Could you check a few things on this model? Use its own coordinates, in mm. Round coordinates to 2 decimals unless told otherwise and drop trailing zeros. Order: outer loops, then holes, each group sorted by start corner. A loop starts at its lowest first (then second) coordinate and runs counter-clockwise, first axis right, second up. Notation, with made-up numbers: (85, 22) - (118, 22) arc R12 ccw to (118, 38) - close; hole circle Ø2 at (43, 76). An arc over 180 degrees is marked (long way). Return JSON: item names as keys, results as strings. Group by question number.
from build123d import *

# Parameters (mm, degrees)
SKETCH_1_W             = 70
SKETCH_1_H             = 310
EXTRUDE_1_DEPTH        = 12
SKETCH_2_R             = 13
CUT_EXTRUDE_1_DEPTH    = 160.354949719
PATTERN_LINEAR_1_COUNT = 4
PATTERN_LINEAR_1_PITCH = 80


with BuildPart() as part:
    # 草图1 → 凸台-拉伸1 (new body)
    with BuildSketch(Plane.XY):
        Rectangle(SKETCH_1_W, SKETCH_1_H)
    extrude(amount=EXTRUDE_1_DEPTH)

    # 草图2 → 切除-拉伸1 (cut, through all)
    with BuildSketch(Plane.XY.offset(12)):
        with Locations((0, 120)):
            Circle(SKETCH_2_R)
    cut_extrude_1 = extrude(amount=-CUT_EXTRUDE_1_DEPTH, mode=Mode.SUBTRACT)

    # 阵列(线性)1: 切除-拉伸1 ×4
    with Locations(*[(0, -i * PATTERN_LINEAR_1_PITCH, 0) for i in range(1, PATTERN_LINEAR_1_COUNT)]):
        add(cut_extrude_1, mode=Mode.SUBTRACT)


solid = part.part
1) If I drill on line 1 along Y through (x, z) = (0, 9.5); line 2 along Y through (x, z) = (3.5, 5.5); line 3 along X through (y, z) = (113.5, 10.75), over which ranges is the centre line in solid material (lowest first)? Write a range as from..to.
2) I want a section at C-C, the plane z = 10. List the corners of the cut face in (x, y) for me.
3) We'd pull the mould along X, two halves only. Please class faces 1 (the flat face through (0, -155, 6)), 2 (the cylindrical face through (-2.82, -132.69, 6.08)), 3 (the flat face through (35, -2, 6)): +X half, -X half, draft (parallel to the pull), parting line (faces both ways), or undercut.
4) I want a section at A-A, the plane y = 40. List the corners of the cut face in (x, z) for me.
5) I want a section at B-B, the plane x = 0. List the corners of the cut face in (y, z) for me, plus the area to 3 significant figures.
Outcome:
{
 "1": {"line 1": "-155..-133, -107..-53, -27..27, 53..107, 133..155", "line 2": "-155..-132.52, -107.48..-52.52, -27.48..27.48, 52.52..107.48, 132.52..155", "line 3": "-35..-11.26, 11.26..35"},
 "2": {"outline": "(-35, -155) - (35, -155) - (35, 155) - (-35, 155) - close; hole circle Ø26 at (0, -120); hole circle Ø26 at (0, -40); hole circle Ø26 at (0, 40); hole circle Ø26 at (0, 120)"},
 "3": {"face 1": "draft", "face 2": "undercut", "face 3": "+X half"},
 "4": {"outline": "(-35, 0) - (-13, 0) - (-13, 12) - (-35, 12) - close; (13, 0) - (35, 0) - (35, 12) - (13, 12) - close"},
 "5": {"outline": "(-155, 0) - (-133, 0) - (-133, 12) - (-155, 12) - close; (-107, 0) - (-53, 0) - (-53, 12) - (-107, 12) - close; (-27, 0) - (27, 0) - (27, 12) - (-27, 12) - close; (53, 0) - (107, 0) - (107, 12) - (53, 12) - close; (133, 0) - (155, 0) - (155, 12) - (133, 12) - close", "area": "2,470 mm^2"}
}
